Input: part model. Units: mm. Frame: model coordinates. Coordinates: 2 decimals unless noted, no trailing zeros. Write each loop counter-clockwise with the first axis right and the second up, starting at its lowest first coordinate (ties: lowest second). Pieces come first, ordered by that corner, then holes. Notation, with made-up numbers: M 70,50 L 124,50 A20 cw 124,84 Z; hole C 10.25,78.5 d7. An arc over 180 degrees is marked long. Use one line per item in the form item = value.
Autodesk Inventor part; units mm, degrees
ref_plane "YZ Plane" through (0, 0, 0) normal (1, 0, 0) x (0, 1, 0)
ref_plane "XZ Plane" through (0, 0, 0) normal (0, 1, 0) x (-1, 0, 0)
ref_plane "XY Plane" through (0, 0, 0) normal (0, 0, 1) x (1, 0, 0)
sketch "Sketch1" plane through (0, 0, 0) normal (0, 0, 1) x (1, 0, 0)
  line L0 (0, 0) -> (50, 0)
  line L1 (50, 0) -> (50, 20)
  line L2 (50, 20) -> (0, 20)
  line L3 (0, 20) -> (0, 0)
  dimension "d0" = 50
  dimension "d1" = 20
extrude "Extrusion1" add sketch "Sketch1" along normal blind 3
sketch "Sketch2" plane through (0, 0, 0) normal (0, -1, 0) x (1, 0, 0)
  line L0 (0, 0) -> (50, 0)
  line L1 (0, 0) -> (50, 0)
  line L2 (50, 0) -> (50, 40)
  line L3 (50, 40) -> (0, 40)
  line L4 (0, 40) -> (0, 0)
  line L5 (50, 0) -> (50, 3)
  dimension "d4" = 40
extrude "Extrusion2" add sketch "Sketch2" along normal blind 3
(1) Line query: probe 1 along Z at (x, y) = (43, 16.5); probe 2 along Y at (x, z) = (41, 33.5). Output: solid intervals per line, ascending.
Computed:
probe_1 = 0 to 3
probe_2 = -3 to 0
(2) Section query C-C on y = 13.5. Return the cut outline in (x, z), plus the area to 3 significant figures.
Computed:
outline = M 0,0 L 50,0 L 50,3 L 0,3 Z
area = 150 mm^2
(3) Pull-direction query (Z, two-part tool) for faces 1 (the flat face through (25, 0, 22)), 2 (the flat face through (25, 10, 3)), 3 (the flat face through (25, 9, 0)); classes: pulls with the +Z half, pulls with the -Z half, needs draft (parallel to the pull), parting line crosses it, or undercut.
Computed:
face_1 = needs draft
face_2 = pulls with the +Z half
face_3 = pulls with the -Z half
(4) First-contact query: pin 1 Ø5 at (x, y) = (43.5, 14.5) entering from +Z; pin 2 Ø4 at (x, y) = (17, 16) entering from -Z; pin 3 Ø2 at (x, z) = (9.5, 31.5) entering from +Y. Flat tips, straight axial feed; report the tip coordinate or a pass-through.
Computed:
pin_1 = 3
pin_2 = 0
pin_3 = 0
(5) Section query A-A on x = 19. Return the cut outline in (y, z), plus the area to 3 significant figures.
Computed:
outline = M -3,0 L 20,0 L 20,3 L 0,3 L 0,40 L -3,40 Z
area = 180 mm^2
(6) Section query B-B on z = 5. Return the cut outline in (x, y).
Computed:
outline = M 0,-3 L 50,-3 L 50,0 L 0,0 Z
